Geometry: final body of the model. Coordinates: model frame, mm. Face numbers are marked on the shaded views. Round coordinates to 2 decimals unless told otherwise and drop trailing zeros. Loops run counter-clockwise (first coordinate to the right, second up) from the corner with the lowest first, then second, coordinate; pieces in that order, holes last. Notation, with made-up numbers: M -9,-19 L 10,-19 A31 ccw 10,6 Z; hole C 60,31 d2. An arc over 180 degrees is marked long. Return JSON: item names as keys, results as strings.
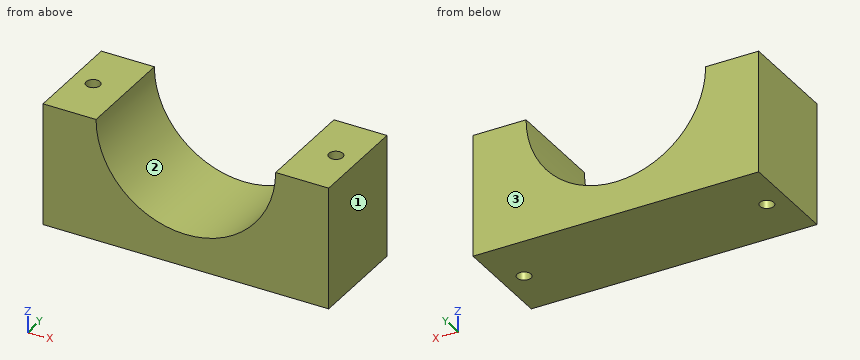
from build123d import *

# Parameters (mm, degrees)
BOSS_EXTRUDE1_DEPTH = 25
SKETCH3_R           = 1.7
BOSS_EXTRUDE2_DEPTH = 30
SKETCH3_2_R         = 1.7
CUT_EXTRUDE1_DEPTH  = 30


with BuildPart() as part:
    # Sketch1 → Boss-Extrude1 (new body)
    with BuildSketch(Plane(origin=(0, 0, 0), x_dir=(1, 0, 0), z_dir=(0, 1, 0))):
        with BuildLine():
            ThreePointArc((27.453920769, 0), (5.453920769, 22), (-16.546079231, 0))
            Line((-16.546079231, 0), (-29.546079231, 0))
            Line((-29.546079231, 0), (-29.546079231, 30))
            Line((-29.546079231, 30), (40.453920769, 30))
            Line((40.453920769, 30), (40.453920769, 0))
            Line((40.453920769, 0), (27.453920769, 0))
        make_face()
    extrude(amount=BOSS_EXTRUDE1_DEPTH)

    # Sketch3 → Boss-Extrude2 (add)
    with BuildSketch(Plane(origin=(0, 0, -30), x_dir=(-1, 0, 0), z_dir=(0, 0, -1))):
        with Locations((-35.073920769, 12.5)):
            Circle(SKETCH3_R)
        with Locations((24.416079231, 12.5)):
            Circle(SKETCH3_R)
    extrude(amount=-BOSS_EXTRUDE2_DEPTH)

    # Sketch3_2 → Cut-Extrude1 (cut)
    with BuildSketch(Plane(origin=(0, 0, -30), x_dir=(-1, 0, 0), z_dir=(0, 0, -1))):
        with Locations((-35.073920769, 12.5)):
            Circle(SKETCH3_2_R)
        with Locations((24.416079231, 12.5)):
            Circle(SKETCH3_2_R)
    extrude(amount=-CUT_EXTRUDE1_DEPTH, mode=Mode.SUBTRACT)


solid = part.part
Q1. Section query B-B (z = -11.5). Output: boundary loops of the cut face in (x, y).
Determined:
{"outline": "M -29.55,0 L -13.3,0 L -13.3,25 L -29.55,25 Z; M 24.21,0 L 40.45,0 L 40.45,25 L 24.21,25 Z; hole C -24.42,12.5 d3.4; hole C 35.07,12.5 d3.4"}
Q2. Material intervals for L1, parallel to Y at x = 35, z = -11.5; L2, parallel to X at y = 13.5, z = -9; L3, parallel to X at y = 5, z = -18.75, sorted ascending.
Determined:
{"L1": "y = 0 to 10.8, 14.2 to 25", "L2": "x = -29.55 to -25.79, -23.04 to -14.62, 25.53 to 33.7, 36.45 to 40.45", "L3": "x = -29.55 to -6.05, 16.96 to 40.45"}
Q3. Pull-direction query (X, two-part tool) for the marked faces 1, 2 and 3; classes: pulls with the +X half, pulls with the -X half, needs draft (parallel to the pull), parting line crosses it, or undercut.
Determined:
{"face 1": "pulls with the +X half", "face 2": "undercut", "face 3": "needs draft"}
Q4. Section query C-C (y = 5.5). Output: boundary loops of the cut face in (x, z).
Determined:
{"outline": "M -29.55,-30 L 40.45,-30 L 40.45,0 L 27.45,0 A22 cw -16.55,0 L -29.55,0 Z"}
Q5. Pin query (flat end, axial travel): pin 1 (2 mm diameter, centred on x = 35.07, y = 12.5, fed in from +Z); pin 2 (8 mm diameter, centred on x = -5, y = 6, fed in from +Z); pin 3 (4 mm diameter, centred on x = 18, y = 22.5, fed in from +Z). Return the tip coordinate at first contact, or that it passes through.
Determined:
{"pin 1": "passes through", "pin 2": "stops at z = -16.59", "pin 3": "stops at z = -16.5"}
Q6. Section query D-D (z = -7). Output: boundary loops of the cut face in (x, y).
Determined:
{"outline": "M -29.55,0 L -15.4,0 L -15.4,25 L -29.55,25 Z; M 26.31,0 L 40.45,0 L 40.45,25 L 26.31,25 Z; hole C -24.42,12.5 d3.4; hole C 35.07,12.5 d3.4"}
Q7. Section query A-A (y = 12.5). Output: boundary loops of the cut face in (x, z), plus the area to 3 significant figures.
Determined:
{"outline": "M -29.55,-30 L -26.12,-30 L -26.12,0 L -29.55,0 Z; M -22.72,-30 L 33.37,-30 L 33.37,0 L 27.45,0 A22 cw -16.55,0 L -22.72,0 Z; M 36.77,-30 L 40.45,-30 L 40.45,0 L 36.77,0 Z", "area": "1,140 mm^2"}
